Can you work these out from the model? Positions are in its coordinate system, mm. Face numbers are marked on the shaded views. A direction names the side the tool comes from. Round coordinates to 2 decimals unless told otherwise and drop trailing zeros. Write each loop counter-clockwise with the first axis right and the second up, starting at its lowest first coordinate (ties: lowest second). Pieces come first, ordered by that corner, then holes. Notation, with made-up numbers: (-23.75, 7) - (20.25, 7) arc R30 ccw to (20.25, 36) - close; hole circle Ø8 at (-37, 68.5). An arc over 180 degrees is marked (long way). One line per item, written item: value. Start each with the question number.
(1) On a 3-axis mill with a long thin cutter (end or side, diameter ignored), from which of +Z, -Z, +X, -X, +Y, -Y can I reach the whole of each face in a straight line? I mean the marked faces 4, 5 and 6. Say none if no direction works.
(2) Thinking about a two-plate mould opening in Y: for the marked faces 1, 2 and 3, which applies, +Y half, -Y half, draft (parallel to the pull), parting line (faces both ways), or undercut?
(3) I want a section at B-B on z = 0. Give the number of separate pieces and of enclosed holes in the cut face, plus the area to 3 significant figures.
(4) If I drill on L1, parallel to Y at x = 6.25, z = -4.5; L2, parallel to Z at x = 5.25, y = 5.5; L3, parallel to Z at x = 6.75, y = 9, over which ranges is the centre line in solid material (lowest first)? Write a range as from..to.
(5) I'm going to push flat-ended pins straight in: pin 1 Ø2.5 at (y, z) = (0, 9.5) entering from -X; pin 2 Ø6 at (x, z) = (9.5, -1.5) entering from -Y; pin 3 Ø10 at (y, z) = (-9, 14.5) entering from +X; pin 4 Ø10 at (y, z) = (0, 0) entering from -X. Where does each tip first touch, or does it pass through?
(6) I want a section at A-A on x = 2.25. List the corners of the cut face in (y, z) for me, plus the area to 3 significant figures.
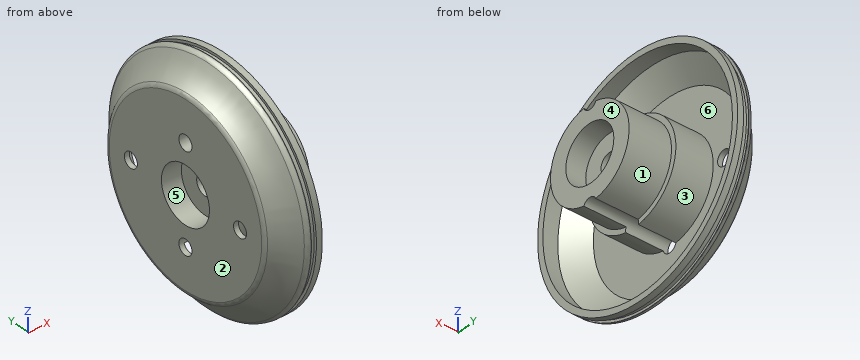
from build123d import *

# Parameters (mm, degrees)
FILLET1_R          = 1
SKETCH3_R          = 1.5
CUT_EXTRUDE2_DEPTH = 37.576222301


with BuildPart() as part:
    # Sketch1 → Revolve1 (revolve)
    with BuildSketch(Plane.XY, mode=Mode.PRIVATE) as revolve1_sk:
        with BuildLine():
            Line((4, 2), (4, 5.5))
            Line((4, 5.5), (0, 5.5))
            Line((0, 5.5), (0, 18))
            ThreePointArc((0, 18), (2.598670777, 20.129792144), (4.5, 22.9))
            Line((4.5, 22.9), (5.2, 22.9))
            Line((5.2, 22.9), (5.2, 22.4))
            Line((5.2, 22.4), (6.2, 22.4))
            Line((6.2, 22.4), (6.2, 22.9))
            Line((6.2, 22.9), (7.4, 22.9))
            Line((7.4, 22.9), (7.4, 21.7))
            Line((7.4, 21.7), (4.4, 21.7))
            Line((4.4, 21.7), (1, 17.446887131))
            Line((1, 17.446887131), (1, 10))
            Line((1, 10), (8.5, 10))
            Line((8.5, 10), (8.5, 9))
            Line((8.5, 9), (17, 9))
            Line((17, 9), (17, 5.5))
            Line((17, 5.5), (13, 5.5))
            Line((13, 5.5), (13, 2))
            Line((13, 2), (4, 2))
        make_face()
    revolve(revolve1_sk.sketch.rotate(Axis((0, 0, 0), (1, 0, 0)), 90), axis=Axis((0, 0, 0), (1, 0, 0)))

    # Fillet1
    fillet1_edges = [part.edges().sort_by_distance(p)[0] for p in [
        (4.5, 0, -22.9),
        (0, 0, -18),
    ]]
    fillet(fillet1_edges, radius=FILLET1_R)

    # Sketch3 → Cut-Extrude2 (cut, through all)
    with BuildSketch(Plane.ZY):
        with Locations(Location((-9.5, 0, 0), (0, 0, 270))):
            Circle(SKETCH3_R)
        with Locations(Location((0, 12.5, 0), (0, 0, 270))):
            Circle(SKETCH3_R)
        with Locations(Location((9.5, 0, 0), (0, 0, 270))):
            Circle(SKETCH3_R)
        with Locations(Location((0, -12.5, 0), (0, 0, 270))):
            Circle(SKETCH3_R)
    extrude(amount=-CUT_EXTRUDE2_DEPTH, mode=Mode.SUBTRACT)


solid = part.part
Established:
1. face 4: +Z, -Z, +X, +Y, -Y
1. face 5: -X
1. face 6: +X
2. face 1: +Y half
2. face 2: draft
2. face 3: undercut
3. separate pieces: 4
3. enclosed holes: 0
3. area: 221 mm2
4. L1: -22.45..-21.23, -8.93..8.93, 21.23..22.45
4. L2: -21.71..-20.99, -8.35..8.35, 20.99..21.71
4. L3: -21.06..-19.75, -4.36..4.36, 19.75..21.06
5. pin 1: through
5. pin 2: y = -22.9
5. pin 3: x = 7.4
5. pin 4: x = 4
6. outline: circle Ø39.53 at (0, 0); (-1.45, -9.89) arc R1.5 cw (long way) to (1.45, -9.89) arc R10 ccw to (1.45, 9.89) arc R1.5 cw (long way) to (-1.45, 9.89) arc R10 ccw to start; hole circle Ø38.02 at (0, 0); hole circle Ø11 at (0, 0)
6. area: 301 mm2
